from build123d import *

# Parameters (mm, degrees)
BOSS_EXTRUDE1_DEPTH = 20
EXTRUDE_THIN3_DEPTH = 21
SKETCH3_R           = 2.75
CUT_EXTRUDE1_DEPTH  = 73.35515227
FILLET2_R           = 3


with BuildPart() as part:
    # Sketch1 → Boss-Extrude1 (new body)
    with BuildSketch(Plane(origin=(0, 0, 0), x_dir=(1, 0, 0), z_dir=(0, 1, 0))):
        Polygon((-32.516534914, -1.83981797), (-32.516534914, 13.66018203), (67.483465086, 13.66018203), (67.483465086, -1.83981797), (50.983465086, -1.83981797), (50.983465086, 1.63642231), (50.983465086, 6.16018203), (48.983465086, 6.16018203), (48.983465086, 0.16018203), (34.983465086, 0.16018203), (34.983465086, 6.16018203), (32.983465086, 6.16018203), (32.983465086, 1.63642231), (32.983465086, -1.83981797), (1.983465086, -1.83981797), (1.983465086, 1.63642231), (1.983465086, 6.16018203), (-0.016534914, 6.16018203), (-0.016534914, 0.16018203), (-14.016534914, 0.16018203), (-14.016534914, 6.16018203), (-16.016534914, 6.16018203), (-16.016534914, 1.63642231), (-16.016534914, -1.83981797), align=None)
    extrude(amount=BOSS_EXTRUDE1_DEPTH)

    # Sketch2 → Extrude-Thin3 (add)
    with BuildSketch(Plane.XZ):
        Polygon((-19.016534914, 1.83981797), (-19.016534914, -13.66018203), (4.983465086, -13.66018203), (4.983465086, 1.83981797), (1.983465086, 1.83981797), (1.983465086, -10.66018203), (-16.016534914, -10.66018203), (-16.016534914, 1.83981797), align=None)
        Polygon((50.983465086, 1.83981797), (50.983465086, -10.66018203), (32.983465086, -10.66018203), (32.983465086, 1.83981797), (29.983465086, 1.83981797), (29.983465086, -13.66018203), (53.983465086, -13.66018203), (53.983465086, 1.83981797), align=None)
    extrude(amount=EXTRUDE_THIN3_DEPTH)

    # Sketch3 → Cut-Extrude1 (cut, through all)
    with BuildSketch(Plane(origin=(0, 0, -13.66018203), x_dir=(-1, 0, 0), z_dir=(0, 0, -1))):
        with Locations((24.516534914, 10)):
            Circle(SKETCH3_R)
        with Locations((-59.483465086, 10)):
            Circle(SKETCH3_R)
        with Locations((-17.483465086, 10)):
            Circle(SKETCH3_R)
    extrude(amount=-CUT_EXTRUDE1_DEPTH, mode=Mode.SUBTRACT)

    # Fillet2
    fillet2_edges = [part.edges().sort_by_distance(p)[0] for p in [
        (17.483465086, 0, -13.66018203),
        (29.983465086, -10.5, -13.66018203),
        (53.983465086, -10.5, -13.66018203),
        (60.733465086, 0, -13.66018203),
        (67.483465086, 0, -5.91018203),
        (67.483465086, 10, -13.66018203),
        (67.483465086, 20, -5.91018203),
        (17.483465086, 20, -13.66018203),
        (-32.516534914, 20, -5.91018203),
        (-32.516534914, 0, -5.91018203),
        (-19.016534914, 0, -5.91018203),
        (4.983465086, -10.5, -13.66018203),
        (-19.016534914, -10.5, -13.66018203),
        (-25.766534914, 0, -13.66018203),
        (-32.516534914, 10, -13.66018203),
        (53.983465086, 0, -5.91018203),
    ]]
    fillet(fillet2_edges, radius=FILLET2_R)


solid = part.part
Geometry check sheet. Reference: the model listing, model coordinates, mm. A direction names the side the tool comes from. Round coordinates to 2 decimals unless told otherwise and drop trailing zeros. Loops run counter-clockwise (first coordinate to the right, second up) from the corner with the lowest first, then second, coordinate; pieces in that order, holes last. Notation, with made-up numbers: (-24.75, 35) - (-8.75, 35) arc R9 ccw to (-8.75, 51) - close; hole circle Ø1 at (75, -18.5). An arc over 180 degrees is marked (long way). Answer as CSV lines item,"result".
(1) Cross-section at D-D, the plane x = -12.5. Enter the section's corners in (y, z).
Output values:
outline,"(-21, -13.66) - (17, -13.66) arc R3 ccw to (20, -10.66) - (20, -0.16) - (0, -0.16) - (0, -10.66) - (-21, -10.66) - close"
(2) Material ranges on line 1 along X through (y, z) = (-15, -8.75); line 2 along X through (y, z) = (11, 1.25); line 3 along X through (y, z) = (-19, -11), recorded low to high.
Output values:
line 1,"x = -19.02 to -16.02, 1.98 to 4.98, 29.98 to 32.98, 50.98 to 53.98"
line 2,"x = -32.52 to -27.08, -21.95 to -16.02, 1.98 to 14.92, 20.05 to 32.98, 50.98 to 56.92, 62.05 to 67.48"
line 3,"x = -19 to 4.96, 30 to 53.96"
(3) Cross-section at A-A, the plane y = -5. Enter the section's corners in (x, z), and give its area (3 significant figures).
Output values:
outline,"(-19.02, -10.66) arc R3 ccw to (-16.02, -13.66) - (1.98, -13.66) arc R3 ccw to (4.98, -10.66) - (4.98, 1.84) - (1.98, 1.84) - (1.98, -10.66) - (-16.02, -10.66) - (-16.02, 1.84) - (-19.02, 1.84) - close; (29.98, -10.66) arc R3 ccw to (32.98, -13.66) - (50.98, -13.66) arc R3 ccw to (53.98, -10.66) - (53.98, 1.84) - (50.98, 1.84) - (50.98, -10.66) - (32.98, -10.66) - (32.98, 1.84) - (29.98, 1.84) - close"
area,"286 mm²"
(4) Release check for a two-part mould opening along X. For faces 1 (the face through (-31.614, 0.855, -4.498)), 2 (the face through (61, 0, -4)), 3 (the face through (-7, -10, -10.66)) record: released by +X, released by -X, zero draft, split by the parting line, or undercut.
Output values:
face 1,"released by -X"
face 2,"zero draft"
face 3,"undercut"
(5) Set-up check for faces 4 (the face through (-25.7, 0.9, -12.8)), 5 (the face through (60.8, 0.9, -12.8)), 6 (the face through (-0.017, 10, -3)): record each of +Z, -Z, +X, -X, +Y, -Y from which the full face is reachable in a straight line by a thin tool's end or side.
Output values:
face 4,"-Z, -X, -Y"
face 5,"-Z, +X, -Y"
face 6,"+Z, +Y, -Y"
(6) Depth check by flat-ended pin: pin 1 Ø15.5 at (x, y) = (44.5, 7.5) entering from +Z; pin 2 Ø6 at (x, z) = (21.5, -4) entering from -Y; pin 3 Ø14.5 at (x, y) = (-5.5, -11) entering from +Z; pin 4 Ø1 at (y, z) = (-7, -6.5) entering from -X. Enter the tip coordinate at first touch or a pass-through.
Output values:
pin 1,"stops at z = 1.84"
pin 2,"stops at y = 0"
pin 3,"stops at z = -10.66"
pin 4,"stops at x = -19.02"
(7) Cross-section at B-B, the plane y = 10. Give the number of separate pieces and of enclosed holes in the cut face, and give its area (3 significant figures).
Output values:
separate pieces,"4"
enclosed holes,"0"
area,"1,170 mm²"
